from build123d import *

# Parameters (mm, degrees)
SKETCH1_R           = 10.5
SKETCH1_R_2         = 1.5
SKETCH1_W           = 8
SKETCH1_H           = 40
SKETCH1_R_3         = 17.5
BOSS_EXTRUDE1_DEPTH = 3
CUT_EXTRUDE1_REACH  = 140.687
SKETCH2_R           = 2
CUT_EXTRUDE2_REACH  = 140.687
SKETCH3_R           = 2


with BuildPart() as part:
    # Sketch1 → Boss-Extrude1 (new body)
    # profile 1 of 2: a face of its own
    with BuildSketch(Plane.XY):
        with BuildLine():
            ThreePointArc((-60, 0), (-52.867640737, 28.372743309), (-33.166247904, 50))
            Line((-33.166247904, 50), (-60, 50))
            Line((-60, 50), (-60, 0))
        make_face()
    # profile 2 of 2: a face of its own
    with BuildSketch(Plane.XY):
        with BuildLine():
            ThreePointArc((0, 60), (-17.320508076, 57.445626465), (-33.166247904, 50))
            ThreePointArc((-33.166247904, 50), (-52.867640737, 28.372743309), (-60, 0))
            ThreePointArc((-60, 0), (-15.529142706, -57.955549577), (51.961524227, -30))
            Line((51.961524227, -30), (56.568542495, -30))
            Line((56.568542495, -30), (90, -30))
            Line((90, -30), (90, -10.355339059))
            Line((90, -10.355339059), (117.67766953, 17.32233047))
            ThreePointArc((117.67766953, 17.32233047), (123.096988313, 44.567085809), (100, 60))
            Line((100, 60), (0, 60))
        make_face()
        Circle(SKETCH1_R, mode=Mode.SUBTRACT)
        with Locations((69, -26)):
            Circle(SKETCH1_R_2, mode=Mode.SUBTRACT)
        with Locations((76, 0)):
            Rectangle(SKETCH1_W, SKETCH1_H, mode=Mode.SUBTRACT)
        with Locations((83, -26)):
            Circle(SKETCH1_R_2, mode=Mode.SUBTRACT)
        with Locations((100, 35)):
            Circle(SKETCH1_R_3, mode=Mode.SUBTRACT)
    extrude(amount=BOSS_EXTRUDE1_DEPTH)

    # Sketch2 → Cut-Extrude1 (cut, up to next)
    with BuildSketch(Plane.XY.offset(3), mode=Mode.PRIVATE) as cut_extrude1_sk1:
        with Locations((60, 45)):
            Circle(SKETCH2_R)
    cut_extrude1_tool1 = extrude(cut_extrude1_sk1.sketch, amount=-CUT_EXTRUDE1_REACH, mode=Mode.PRIVATE) & part.part
    add(cut_extrude1_tool1.solids().sort_by_distance((60, 45, 3))[0], mode=Mode.SUBTRACT)

    # Sketch3 → Cut-Extrude2 (cut, up to next)
    with BuildSketch(Plane.XY.offset(3), mode=Mode.PRIVATE) as cut_extrude2_sk1:
        with Locations((100, 10)):
            Circle(SKETCH3_R)
    cut_extrude2_tool1 = extrude(cut_extrude2_sk1.sketch, amount=-CUT_EXTRUDE2_REACH, mode=Mode.PRIVATE) & part.part
    # Sketch3 → Cut-Extrude2 (cut, up to next)
    with BuildSketch(Plane.XY.offset(3), mode=Mode.PRIVATE) as cut_extrude2_sk2:
        with Locations((75, 35)):
            Circle(SKETCH3_R)
    cut_extrude2_tool2 = extrude(cut_extrude2_sk2.sketch, amount=-CUT_EXTRUDE2_REACH, mode=Mode.PRIVATE) & part.part
    # Sketch3 → Cut-Extrude2 (cut, up to next)
    with BuildSketch(Plane.XY.offset(3), mode=Mode.PRIVATE) as cut_extrude2_sk3:
        with Locations((115.0260191, 50.0260191)):
            Circle(SKETCH3_R)
    cut_extrude2_tool3 = extrude(cut_extrude2_sk3.sketch, amount=-CUT_EXTRUDE2_REACH, mode=Mode.PRIVATE) & part.part
    add(cut_extrude2_tool1.solids().sort_by_distance((100, 10, 3))[0], mode=Mode.SUBTRACT)
    add(cut_extrude2_tool2.solids().sort_by_distance((75, 35, 3))[0], mode=Mode.SUBTRACT)
    add(cut_extrude2_tool3.solids().sort_by_distance((115.026019, 50.026019, 3))[0], mode=Mode.SUBTRACT)


solid = part.part
Verification items for the finished model (mm, model axes). Give positions to 0.01 mm unless a question says otherwise; leave off trailing zeros. Write each loop counter-clockwise with the first axis right and the second up, starting at its lowest first coordinate (ties: lowest second). Pieces come first, ordered by that corner, then holes. Notation, with made-up numbers: M -28.5,61.5 L 1.5,61.5 A19 ccw 1.5,96.5 Z; hole C 47.25,4 d2. An arc over 180 degrees is marked long. Put each result on its own line as item: value. Start each with the question number.
1. Section check D-D (y = -36). Record the cut outline in (x, z).
2. Section check A-A (x = 75). Record the cut outline in (y, z).
3. Section check C-C (z = 0.8). Give the number of separate pieces and of enclosed holes in the cut face, and give its area (3 significant figures).
4. Draft check along X on faces 1 (the face through (103.645, 3.29, 1.479)), 2 (the face through (-16.59, -57.66, 1.48)), 3 (the face through (11, 14, 3)), 4 (the face through (101.908, 10.601, 1.521)). Enter one of: +X half, -X half, draft (parallel to the pull), parting line (faces both ways), or undercut.
5. Scan lines: line 1 along Y through (x, z) = (75, 0.85); line 2 along Y through (x, z) = (0, 1.1); line 3 along Y through (x, z) = (114.5, 1.65). Record each from-to range of solid material in increasing order. Write a range as [from, to].
6. Go/stop test with flat-tipped pins: pin 1 Ø1.5 at (x, z) = (95, 0.5) entering from -Y; pin 2 Ø1.5 at (x, z) = (-15, 2) entering from +Y; pin 3 Ø0.9 at (x, z) = (75, 1) entering from -Y; pin 4 Ø5 at (x, y) = (83, -26) entering from +Z. Record where each tip stops, or that it passes through.
7. Section check B-B (y = 39.5). Record the cut outline in (x, z), and give its area (3 significant figures).
Answer list:
1. outline: M -48,0 L 48,0 L 48,3 L -48,3 Z
2. outline: M -30,0 L -20,0 L -20,3 L -30,3 Z; M 20,0 L 33,0 L 33,3 L 20,3 Z; M 37,0 L 60,0 L 60,3 L 37,3 Z
3. separate pieces: 1
3. enclosed holes: 9
3. area: 15,300 mm2
4. face 1: +X half
4. face 2: parting line
4. face 3: draft
4. face 4: undercut
5. line 1: [-30, -20], [20, 33], [37, 60]
5. line 2: [-60, -10.5], [10.5, 60]
5. line 3: [14.14, 25.2], [44.8, 48.1], [51.96, 55.37]
6. pin 1: y = -6.11
6. pin 2: y = 58.28
6. pin 3: y = -30
6. pin 4: z = 3
7. outline: M -60,0 L 83.09,0 L 83.09,3 L -60,3 Z; M 116.91,0 L 124.59,0 L 124.59,3 L 116.91,3 Z
7. area: 452 mm2
